```python
from build123d import *

# Parameters (mm, degrees)
SKETCH1_R           = 11.1
BOSS_EXTRUDE1_DEPTH = 12
BOSS_EXTRUDE2_START = -2
SKETCH3_R           = 11.1
BOSS_EXTRUDE2_DEPTH = 2
SKETCH4_W           = 55
SKETCH4_H           = 5
BOSS_EXTRUDE3_DEPTH = 20
SKETCH5_R           = 2.6
CUT_EXTRUDE1_DEPTH  = 55.428852643
CHAMFER1_SIZE       = 8


with BuildPart() as part:
    # Sketch1 → Boss-Extrude1 (new body)
    with BuildSketch(Plane(origin=(0, 0, 0), x_dir=(1, 0, 0), z_dir=(0, 1, 0))):
        with BuildLine():
            Line((-17.5, 0), (-17.5, -25))
            Line((-17.5, -25), (17.5, -25))
            Line((17.5, -25), (17.5, 0))
            ThreePointArc((17.5, 0), (0, 17.5), (-17.5, 0))
        make_face()
        with Locations(Location((0, 0, 0), (0, 0, 270))):
            Circle(SKETCH1_R, mode=Mode.SUBTRACT)
    extrude(amount=BOSS_EXTRUDE1_DEPTH)

    # Sketch3 → Boss-Extrude2 (add)
    with BuildSketch(Plane(origin=(0, 12, 0), x_dir=(1, 0, 0), z_dir=(0, 1, 0)).offset(BOSS_EXTRUDE2_START)):
        with Locations(Location((0, 0, 0), (0, 0, 270))):
            Circle(SKETCH3_R)
    extrude(amount=BOSS_EXTRUDE2_DEPTH)

    # Sketch4 → Boss-Extrude3 (add)
    with BuildSketch(Plane(origin=(0, 0, 0), x_dir=(1, 0, 0), z_dir=(0, 1, 0))):
        with Locations((0, -27.5)):
            Rectangle(SKETCH4_W, SKETCH4_H)
    extrude(amount=BOSS_EXTRUDE3_DEPTH)

    # Sketch5 → Cut-Extrude1 (cut, through all)
    with BuildSketch(Plane(origin=(0, 0, 25), x_dir=(-1, 0, 0), z_dir=(0, 0, -1))):
        with Locations((22.5, 10)):
            Circle(SKETCH5_R)
        with Locations((-22.5, 10)):
            Circle(SKETCH5_R)
    extrude(amount=-CUT_EXTRUDE1_DEPTH, mode=Mode.SUBTRACT)

    # Chamfer1
    chamfer1_edges = [part.edges().sort_by_distance(p)[0] for p in [
        (0, 12, 25),
    ]]
    chamfer(chamfer1_edges, length=CHAMFER1_SIZE - 0.0001)  # a hair under: the kernel refuses the full size


solid = part.part
```
Check sheet for the modelled part. Datum: model origin and axes. Units: mm. A direction names the side the tool comes from. Give positions to 0.01 mm unless a question says otherwise; leave off trailing zeros. Order: outer loops, then holes, each group sorted by start corner. A loop starts at its lowest first (then second) coordinate and runs counter-clockwise, first axis right, second up. Notation, with made-up numbers: (21, -15) -> (44, -15) arc R31 ccw to (44, 22) -> close; hole circle Ø11 at (3.25, 15). An arc over 180 degrees is marked (long way). Use CSV: the item, a comma, the result in double quotes. Start each with the question number.
1) Sectioned sample at B-B, the plane x = 22.5. Record the boundary of the cut face in (y, z).
2) Sectioned sample at A-A, the plane y = 6.5. Record the boundary of the cut face in (x, z), plus the area to 3 significant figures.
3) Material ranges on line 1 (X direction, y = 10.5, z = 27.5); line 2 (X direction, y = 2.75, z = 0); line 3 (Y direction, x = -5, z = -15), recorded low to high. Write a range as from..to.
4) Mould release check, pull along Y, two halves, no side actions. Record for faces 1 (the face through (0, 20, 27)), 2 (the face through (21.3, 7.693, 27.465)), 3 (the face through (-27.5, 10, 28)), 4 (the face through (0, 0, 16)): released by +Y, released by -Y, zero draft, split by the parting line, or undercut.
5) Go/stop test with flat-tipped pins: P1, Ø10, axis at y = 6.5, z = 8.5, coming from the +X side; P2, Ø12, axis at x = -5, y = 8, coming from the -Z side; P3, Ø10, axis at x = -8.5, z = 6, coming from the +Y side; P4, Ø6, axis at x = -22, y = 5.5, coming from the -Z side. Record where each tip stops, or that it passes through.
6) Sectioned sample at D-D, the plane z = -10. Record the boundary of the cut face in (x, y).
7) Set-up check for faces 5 (the face through (-19, 10, 25)), 6 (the face through (0, 12, 0)), 7 (the face through (17.5, 8, 13)), 8 (the face through (-17.5, 5, 12)), 9 (the face through (9.36, 4.93, 5.97)): record each of +Z, -Z, +X, -X, +Y, -Y from which the full face is reachable in a straight line by a thin tool's end or side.
Recorded:
1,outline,"(0, 25) -> (7.4, 25) -> (7.4, 30) -> (0, 30) -> close; (12.6, 25) -> (20, 25) -> (20, 30) -> (12.6, 30) -> close"
2,outline,"(-27.5, 25) -> (-17.5, 25) -> (-17.5, 0) arc R17.5 ccw to (17.5, 0) -> (17.5, 25) -> (27.5, 25) -> (27.5, 30) -> (-27.5, 30) -> close; hole circle Ø22.2 at (0, 0)"
2,area,"1,240 mm2"
3,line 1,"-27.5..-25.05, -19.95..19.95, 25.05..27.5"
3,line 2,"-17.5..-11.1, 11.1..17.5"
3,line 3,"0..12"
4,face 1,"released by +Y"
4,face 2,"undercut"
4,face 3,"zero draft"
4,face 4,"released by -Y"
5,P1,"x = 17.5"
5,P2,"z = -17.5"
5,P3,"y = 12"
5,P4,"z = 25"
6,outline,"(-14.36, 0) -> (-4.82, 0) -> (-4.82, 10) -> (4.82, 10) -> (4.82, 0) -> (14.36, 0) -> (14.36, 12) -> (-14.36, 12) -> close"
7,face 5,"-Z, +Y, -Y"
7,face 6,"-Z, +X, -X, +Y"
7,face 7,"-Z, +X, +Y, -Y"
7,face 8,"-Z, -X, +Y, -Y"
7,face 9,"-Y"
